Can you work these out from the model? Positions are in its coordinate system, mm. Face numbers are marked on the shaded views. A direction names the side the tool comes from. Give positions to 0.01 mm unless a question says otherwise; leave off trailing zeros. Loops run counter-clockwise (first coordinate to the right, second up) from the corner with the lowest first, then second, coordinate; pieces in that order, holes last. Notation, with made-up numbers: (63.5, -21) - (97.5, -21) arc R11 cw to (97.5, -14) - close; hole circle Ø7 at (47.25, 29.25). An arc over 180 degrees is marked (long way). Use a Markdown table: item, result. Add a question column.
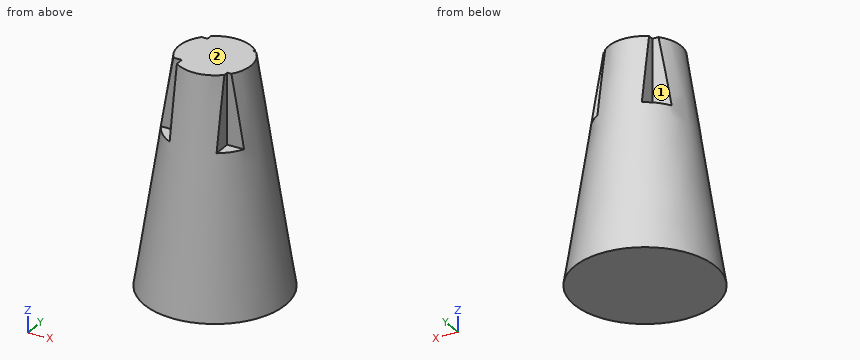
```python
from build123d import *

# Parameters (mm, degrees)
F3_W     = 2.124586
F3_H     = 2.646484
F3_W_2   = 2.326301
F3_H_2   = 2.416364
F3_W_3   = 3.771314
F3_H_3   = 3.010656
F3_W_4   = 3.903168
F3_H_4   = 2.436567
F4_DEPTH = 7.62


with BuildPart() as f1:
    # F0 (on Front) → F1 (revolve)
    with BuildSketch(Plane.XZ):
        Polygon((0, 24.31952), (0, 0), (7.62, 0), (3.901527, 24.31952), align=None)
    revolve(axis=Axis((0, 0, 12.15976), (0, 0, 1)))

    # F3 (on offset) → F4 (cut)
    with BuildSketch(Plane.XY.offset(24.31952)):
        with Locations((3.723198, -3.671215)):
            Rectangle(F3_W, F3_H)
        with Locations((3.787343, 3.782073)):
            Rectangle(F3_W_2, F3_H_2)
        with Locations((-4.159726, -3.779338)):
            Rectangle(F3_W_3, F3_H_3)
        with Locations((-4.225653, 3.792174)):
            Rectangle(F3_W_4, F3_H_4)
    extrude(amount=-F4_DEPTH, mode=Mode.SUBTRACT)


solid = f1.part
```
1. Suppose I cut it at B-B (x = 0). List the corners of the cut face in (y, z) for me.
2. On a 3-axis mill with a long thin cutter (end or side, diameter ignored), from which of +Z, -Z, +X, -X, +Y, -Y can I reach the whole of each face in a straight line? I mean the marked faces 1 and 2. Say none if no direction works.
3. Please list where these lines run through material, in increasing order: line 1 along Z through (x, y) = (4, -2.75); line 2 along Y through (x, z) = (-3, 17); line 3 along Y through (x, z) = (-1.25, 13.25). Write a range as [from, to].
4. Suppose I cut it at A-A (z = 20.75). List the corners of the cut face in (x, y) for me.
5. Suppose I cut it at D-D (z = 14.75). List the corners of the cut face in (x, y) for me, and give its area (3 significant figures).
6. Will these pins go through, and if not, where does the flat tip stop? P1, Ø0.9, axis at x = 3.5, y = -3, coming from the +Z side; P2, Ø0.7, axis at x = -3, z = 20.5, coming from the -Y side; P3, Ø6, axis at y = -5, z = 15.5, coming from the +X side; P4, Ø4, axis at x = 0, y = 3, coming from the -Z side.
Results below:
| question | item | result |
|---|---|---|
| 1 | outline | (-7.62, 0) - (7.62, 0) - (3.9, 24.32) - (-3.9, 24.32) - close |
| 2 | face 1 | +Z, -X, +Y |
| 2 | face 2 | +Z, +X, -X, +Y, -Y |
| 3 | line 1 | [0, 16.7] |
| 3 | line 2 | [-2.27, 2.57] |
| 3 | line 3 | [-5.45, 5.45] |
| 4 | outline | (-3.82, -2.27) - (-2.27, -2.27) - (-2.27, -3.82) arc R4.45 ccw to (2.66, -3.56) - (2.66, -2.35) - (3.78, -2.35) arc R4.45 ccw to (3.63, 2.57) - (2.62, 2.57) - (2.62, 3.59) arc R4.45 ccw to (-2.27, 3.82) - (-2.27, 2.57) - (-3.63, 2.57) arc R4.45 ccw to start |
| 5 | outline | circle Ø10.73 at (0, 0) |
| 5 | area | 90.4 mm² |
| 6 | P1 | z = 16.7 |
| 6 | P2 | y = -2.27 |
| 6 | P3 | x = 4.95 |
| 6 | P4 | z = 0 |
